The figure shows three views and two pictorial views of one solid part (mm, origin at its lowest corner). Answer the questions. A direction names the side the tool comes from. Give positions to 0.01 mm unless a question says otherwise; leave off trailing zeros. Loops run counter-clockwise (first coordinate to the right, second up) from the corner with the lowest first, then second, coordinate; pieces in that order, holes last. Notation, with made-up numbers: (-9, 79) - (44, 79) arc R21 cw to (44, 113) - close; hole circle Ø6 at (16, 53.25). An arc over 180 degrees is marked (long way). Write each question's results on one line, items separated by ' | '.
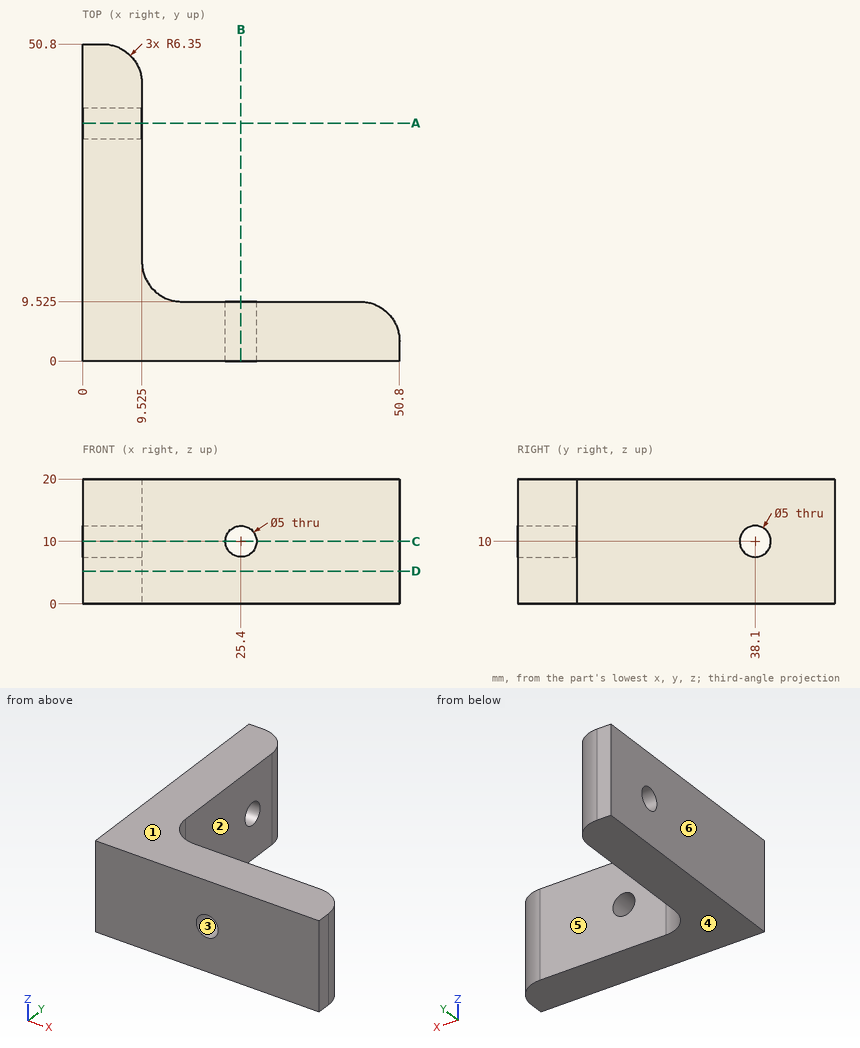
Item 1: A cutting plane is placed at C-C, the plane z = 10. Determine the outline of the cut face in (x, y) (3 decimals).
Values found:
outline: (0, 0) - (22.9, 0) - (22.9, 9.525) - (15.875, 9.525) arc R6.35 cw to (9.525, 15.875) - (9.525, 35.6) - (0, 35.6) - close; (0, 40.6) - (9.525, 40.6) - (9.525, 44.45) arc R6.35 ccw to (3.175, 50.8) - (0, 50.8) - close; (27.9, 0) - (50.8, 0) - (50.8, 3.175) arc R6.35 ccw to (44.45, 9.525) - (27.9, 9.525) - close
Item 2: For a pull along Z with two mould halves and no side action, classify the marked faces 1, 2, 3 and 4 as released by +Z, released by -Z, zero draft, split by the parting line, or undercut.
Values found:
face 1: released by +Z | face 2: zero draft | face 3: undercut | face 4: released by -Z
Item 3: A cutting plane is placed at A-A, the plane y = 38.1. Determine the outline of the cut face in (x, z) (3 decimals).
Values found:
outline: (0, 0) - (9.525, 0) - (9.525, 7.5) - (0, 7.5) - close; (0, 12.5) - (9.525, 12.5) - (9.525, 20) - (0, 20) - close
Item 4: A cutting plane is placed at D-D, the plane z = 5.25. Determine the outline of the cut face in (x, y) (3 decimals).
Values found:
outline: (0, 0) - (50.8, 0) - (50.8, 3.175) arc R6.35 ccw to (44.45, 9.525) - (15.875, 9.525) arc R6.35 cw to (9.525, 15.875) - (9.525, 44.45) arc R6.35 ccw to (3.175, 50.8) - (0, 50.8) - close
Item 5: For the marked faces 5 and 6, determine the directions among +Z, -Z, +X, -X, +Y, -Y from which every point of the face is accessible in a straight line to the end or side of a thin tool.
Values found:
face 5: +Z, -Z, +X, +Y | face 6: +Z, -Z, -X, +Y, -Y
Item 6: Flat-ended cylindrical pins translate along their axes: P1, Ø8, axis at y = 41.5, z = 10.5, coming from the +X side (3 decimals); P2, Ø5, axis at x = 7, z = 8.5, coming from the +Y side; P3, Ø6, axis at x = 33.5, z = 5, coming from the +Y side (3 decimals). Find the tip coordinate at first contact, or state that the pin passes through.
Values found:
P1: stops at x = 9.525 | P2: stops at y = 50.66 | P3: stops at y = 9.525
Item 7: Find the intervals of material crossed by line 1 along Y through (x, z) = (3.5, 10); line 2 along Z through (x, y) = (4, 38); line 3 along X through (y, z) = (30.5, 12.25) (3 decimals), in increasing order. Write a range as [from, to].
Values found:
line 1: y = [0, 35.6], [40.6, 50.79] | line 2: z = [0, 7.5], [12.5, 20] | line 3: x = [0, 9.525]
